Check sheet for the modelled part. Datum: model origin and axes. Units: mm. A direction names the side the tool comes from. Coordinates: 2 decimals unless noted, no trailing zeros. Loops run counter-clockwise (first coordinate to the right, second up) from the corner with the lowest first, then second, coordinate; pieces in that order, holes last. Notation, with made-up numbers: M 10,53.25 L 59,53.25 A12 ccw 59,67.25 Z; hole C 59.5,33 d7. An arc over 180 degrees is marked long. Use CSV: the item, a comma, the result in double quotes. Start each with the question number.
(1) Set-up check for faces 5 (the flat face through (7, 20, 4)), 6 (the flat face through (0, 0, 0)), 7 (the flat face through (7, 83.5, 4)), 8 (the flat face through (-5, 65, -6)), 9 (the flat face through (-3.8, 45.9, 7.5)): record each of +Z, -Z, +X, -X, +Y, -Y from which the full face is reachable in a straight line by a thin tool's end or side.
(2) Section check C-C on y = 8. Record the cut outline in (x, z), and give its area (3 significant figures).
(3) Scan lines: line 1 (Y direction, x = -7, z = 5.75); line 2 (Y direction, x = 4, z = -8.5); line 3 (X direction, y = 42, z = 0.25). Record each from-to range of solid material in increasing order.
(4) Draft check along Y on faces 1 (the cylindrical face through (-9.76, 32.77, -2.17)), 2 (the flat face through (0, 103.5, 0)), 3 (the cylindrical face through (-0.1, 80.5, -6.4)), 4 (the flat face through (0, 66, -4)). Enter one of: pulls with the +Y half, pulls with the -Y half, needs draft (parallel to the pull), parting line crosses it, or undercut.
(5) Section check D-D on z = 5.5. Record the cut outline in (x, y), and give its area (3 significant figures).
(6) Go/stop test with flat-tipped pins: pin 1 Ø1 at (x, y) = (7.5, 62) entering from -Z; pin 2 Ø2.5 at (y, z) = (66.5, -7) entering from -X; pin 3 Ø12 at (y, z) = (11, -1) entering from +X. Record where each tip stops, or that it passes through.
(7) Section check A-A on x = 0. Record the cut outline in (y, z).
(8) Section check B-B on z = 0. Record the cut outline in (x, y), and give its area (3 significant figures).
from build123d import *

# Parameters (mm, degrees)
SKETCH1_R           = 7.5
BOSS_EXTRUDE1_DEPTH = 20
SKETCH2_R           = 10
BOSS_EXTRUDE2_DEPTH = 63.5
SKETCH3_R           = 7.5
BOSS_EXTRUDE3_DEPTH = 20
CUT_EXTRUDE1_DEPTH  = 6
SKETCH5_W           = 1.8
SKETCH5_H           = 1.6


with BuildPart() as part:
    # Sketch1 → Boss-Extrude1 (new body)
    with BuildSketch(Plane(origin=(0, 0, 0), x_dir=(1, 0, 0), z_dir=(0, 1, 0))):
        with Locations(Location((0, 0, 0), (0, 0, 270))):
            Circle(SKETCH1_R)
    extrude(amount=BOSS_EXTRUDE1_DEPTH)

    # Sketch2 → Boss-Extrude2 (add)
    with BuildSketch(Plane(origin=(0, 20, 0), x_dir=(1, 0, 0), z_dir=(0, 1, 0))):
        with Locations(Location((0, 0, 0), (0, 0, 270))):
            Circle(SKETCH2_R)
    extrude(amount=BOSS_EXTRUDE2_DEPTH)

    # Sketch3 → Boss-Extrude3 (add)
    with BuildSketch(Plane(origin=(0, 83.5, 0), x_dir=(1, 0, 0), z_dir=(0, 1, 0))):
        with Locations(Location((0, 0, 0), (0, 0, 270))):
            Circle(SKETCH3_R)
    extrude(amount=BOSS_EXTRUDE3_DEPTH)

    # Sketch4 → Cut-Extrude1 (cut)
    with BuildSketch(Plane(origin=(0, 0, -10), x_dir=(-1, 0, 0), z_dir=(0, 0, -1))):
        with BuildLine():
            Line((-5, 75.5), (-5, 55.5))
            ThreePointArc((-5, 55.5), (0, 50.5), (5, 55.5))
            Line((5, 55.5), (5, 75.5))
            ThreePointArc((5, 75.5), (0, 80.5), (-5, 75.5))
        make_face()
    extrude(amount=-CUT_EXTRUDE1_DEPTH, mode=Mode.SUBTRACT)

    # Sketch5 → Cut-Revolve1 (revolve, cut)
    with BuildSketch(Plane(origin=(0, 0, 0), x_dir=(0, 0, -1), z_dir=(1, 0, 0)), mode=Mode.PRIVATE) as cut_revolve1_sk:
        with Locations((9.1, 46.7)):
            Rectangle(SKETCH5_W, SKETCH5_H)
    revolve(cut_revolve1_sk.sketch.rotate(Axis((0, 103.034047477, 0), (0, -1, 0)), 180), axis=Axis((0, 103.034047477, 0), (0, -1, 0)), mode=Mode.SUBTRACT)


solid = part.part
Outcome:
1,face 5,"-Y"
1,face 6,"+Z, -Z, +X, -X, -Y"
1,face 7,"+Y"
1,face 8,"-Z"
1,face 9,"none"
2,outline,"C 0,0 d15"
2,area,"177 mm²"
3,line 1,"y = 20 to 45.9, 47.5 to 83.5"
3,line 2,"y = 20 to 45.9, 47.5 to 52.5, 78.5 to 83.5"
3,line 3,"x = -10 to 10"
4,face 1,"needs draft"
4,face 2,"pulls with the +Y half"
4,face 3,"undercut"
4,face 4,"undercut"
5,outline,"M -8.35,20 L -5.1,20 L -5.1,0 L 5.1,0 L 5.1,20 L 8.35,20 L 8.35,45.9 L 6.08,45.9 L 6.08,47.5 L 8.35,47.5 L 8.35,83.5 L 5.1,83.5 L 5.1,103.5 L -5.1,103.5 L -5.1,83.5 L -8.35,83.5 L -8.35,47.5 L -6.08,47.5 L -6.08,45.9 L -8.35,45.9 Z"
5,area,"1,460 mm²"
6,pin 1,"stops at z = -7.14"
6,pin 2,"stops at x = -8.18"
6,pin 3,"stops at x = 7.5"
7,outline,"M 0,-7.5 L 20,-7.5 L 20,-10 L 45.9,-10 L 45.9,-8.2 L 47.5,-8.2 L 47.5,-10 L 50.5,-10 L 50.5,-4 L 80.5,-4 L 80.5,-10 L 83.5,-10 L 83.5,-7.5 L 103.5,-7.5 L 103.5,7.5 L 83.5,7.5 L 83.5,10 L 47.5,10 L 47.5,8.2 L 45.9,8.2 L 45.9,10 L 20,10 L 20,7.5 L 0,7.5 Z"
8,outline,"M -10,20 L -7.5,20 L -7.5,0 L 7.5,0 L 7.5,20 L 10,20 L 10,45.9 L 8.2,45.9 L 8.2,47.5 L 10,47.5 L 10,83.5 L 7.5,83.5 L 7.5,103.5 L -7.5,103.5 L -7.5,83.5 L -10,83.5 L -10,47.5 L -8.2,47.5 L -8.2,45.9 L -10,45.9 Z"
8,area,"1,860 mm²"
